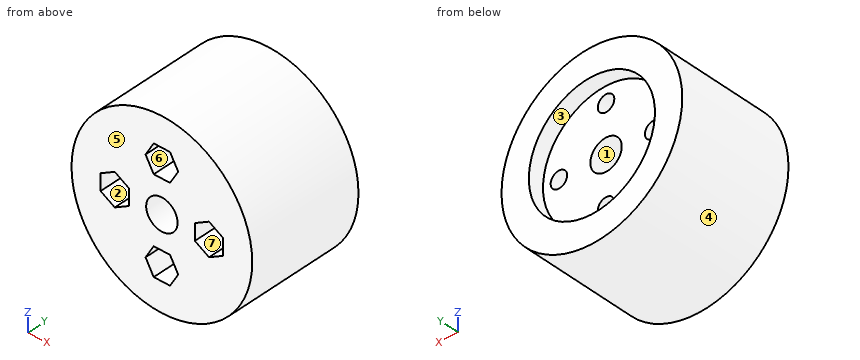
from build123d import *

# Parameters (mm, degrees)
SKETCH1_R           = 23
SKETCH1_R_2         = 4
SKETCH1_R_3         = 2.1
BOSS_EXTRUDE1_DEPTH = 30
SKETCH2_R           = 16.05
CUT_EXTRUDE1_DEPTH  = 4
CUT_EXTRUDE2_DEPTH  = 12


with BuildPart() as part:
    # Sketch1 → Boss-Extrude1 (new body)
    with BuildSketch(Plane(origin=(0, 0, 0), x_dir=(1, 0, 0), z_dir=(0, 1, 0))):
        with Locations(Location((0, 0, 0), (0, 0, 270))):
            Circle(SKETCH1_R)
        with Locations(Location((0, 0, 0), (0, 0, 270))):
            Circle(SKETCH1_R_2, mode=Mode.SUBTRACT)
        with Locations(Location((0, 12, 0), (0, 0, 270))):
            Circle(SKETCH1_R_3, mode=Mode.SUBTRACT)
        with Locations(Location((12, 0, 0), (0, 0, 270))):
            Circle(SKETCH1_R_3, mode=Mode.SUBTRACT)
        with Locations(Location((0, -12, 0), (0, 0, 270))):
            Circle(SKETCH1_R_3, mode=Mode.SUBTRACT)
        with Locations(Location((-12, 0, 0), (0, 0, 270))):
            Circle(SKETCH1_R_3, mode=Mode.SUBTRACT)
    extrude(amount=BOSS_EXTRUDE1_DEPTH)

    # Sketch2 → Cut-Extrude1 (cut)
    with BuildSketch(Plane(origin=(0, 30, 0), x_dir=(1, 0, 0), z_dir=(0, 1, 0))):
        with Locations(Location((0, 0, 0), (0, 0, 270))):
            Circle(SKETCH2_R)
    extrude(amount=-CUT_EXTRUDE1_DEPTH, mode=Mode.SUBTRACT)

    # Sketch3 → Cut-Extrude2 (cut)
    with BuildSketch(Plane.XZ):
        Polygon((12, -4.156921938), (15.6, -2.078460969), (15.6, 2.078460969), (12, 4.156921938), (8.4, 2.078460969), (8.4, -2.078460969), align=None)
        Polygon((4.156921938, 12), (2.078460969, 15.6), (-2.078460969, 15.6), (-4.156921938, 12), (-2.078460969, 8.4), (2.078460969, 8.4), align=None)
        Polygon((-4.156921938, -12), (-2.078460969, -15.6), (2.078460969, -15.6), (4.156921938, -12), (2.078460969, -8.4), (-2.078460969, -8.4), align=None)
        Polygon((-12, 4.156921938), (-15.6, 2.078460969), (-15.6, -2.078460969), (-12, -4.156921938), (-8.4, -2.078460969), (-8.4, 2.078460969), align=None)
    extrude(amount=-CUT_EXTRUDE2_DEPTH, mode=Mode.SUBTRACT)


solid = part.part
Build history of the part. All positions in model axes, mm. Face numbers are marked on the shaded views. A direction names the side the tool comes from. Coordinates: 2 decimals unless noted, no trailing zeros. Order: outer loops, then holes, each group sorted by start corner. A loop starts at its lowest first (then second) coordinate and runs counter-clockwise, first axis right, second up. Notation, with made-up numbers: (-38, -9) - (-4, -9) arc R26 ccw to (-4, 22) - close; hole circle Ø5 at (55, 75.5). An arc over 180 degrees is marked (long way). Write each question's results on one line, items separated by ' | '. Start each with the question number.
Item 1: Flat gauge pins, fed straight in: pin 1 (4 mm diameter, centred on y = 21.5, z = -10, fed in from +X); pin 2 (2 mm diameter, centred on x = 1.5, z = -13, fed in from -Y); pin 3 (12 mm diameter, centred on y = 5, z = -1.5, fed in from +X); pin 4 (1.5 mm diameter, centred on x = -0.5, z = -13, fed in from -Y). Where does each tip first touch, or does it go through?
Item 2: Tool access for the marked faces 1, 2 and 3: list every direction of +Z, -Z, +X, -X, +Y, -Y with a clear straight run to the whole face (end or side of a thin tool).
Item 3: Band-saw the part on D-D on z = -13.5. Write the cut outline in (x, y).
Item 4: Band-saw the part on C-C on y = 2.5. Write the cut outline in (x, z).
Item 5: Band-saw the part on A-A on x = 0. Write the cut outline in (y, z), and give its area (3 significant figures).
Item 6: Mould opens along Z. For the marked faces 4, 5, 6 and 7 say: released by +Z, released by -Z, zero draft, split by the parting line, or undercut.
Item 7: Band-saw the part on B-B on z = 0. Write the cut outline in (x, y), and give its area (3 significant figures).
Item 8: Wall check: probe 1 along X at (y, z) = (13.5, 0); probe 2 along X at (y, z) = (6.5, 3.5); probe 3 along Y at (x, z) = (2.5, -8). Give the ranges that are in metal, low to high. Write a range as [from, to].
Numbers:
1) pin 1: x = 21.56 | pin 2: y = 12 | pin 3: x = 23 | pin 4: through
2) face 1: +Y, -Y | face 2: -Y | face 3: +Y
3) outline: (-18.62, 0) - (-3.29, 0) - (-3.29, 12) - (-1.47, 12) - (-1.47, 26) - (-8.68, 26) - (-8.68, 30) - (-18.62, 30) - close; (1.47, 12) - (3.29, 12) - (3.29, 0) - (18.62, 0) - (18.62, 30) - (8.68, 30) - (8.68, 26) - (1.47, 26) - close
4) outline: circle Ø46 at (0, 0); hole (-15.6, -2.08) - (-12, -4.16) - (-8.4, -2.08) - (-8.4, 2.08) - (-12, 4.16) - (-15.6, 2.08) - close; hole (-4.16, -12) - (-2.08, -15.6) - (2.08, -15.6) - (4.16, -12) - (2.08, -8.4) - (-2.08, -8.4) - close; hole (-4.16, 12) - (-2.08, 8.4) - (2.08, 8.4) - (4.16, 12) - (2.08, 15.6) - (-2.08, 15.6) - close; hole circle Ø8 at (0, 0); hole (8.4, -2.08) - (12, -4.16) - (15.6, -2.08) - (15.6, 2.08) - (12, 4.16) - (8.4, 2.08) - close
5) outline: (0, -23) - (30, -23) - (30, -16.05) - (26, -16.05) - (26, -14.1) - (12, -14.1) - (12, -15.6) - (0, -15.6) - close; (0, -8.4) - (12, -8.4) - (12, -9.9) - (26, -9.9) - (26, -4) - (0, -4) - close; (0, 4) - (26, 4) - (26, 9.9) - (12, 9.9) - (12, 8.4) - (0, 8.4) - close; (0, 15.6) - (12, 15.6) - (12, 14.1) - (26, 14.1) - (26, 16.05) - (30, 16.05) - (30, 23) - (0, 23) - close | area: 753 mm^2
6) face 4: split by the parting line | face 5: zero draft | face 6: undercut | face 7: undercut
7) outline: (-23, 0) - (-15.6, 0) - (-15.6, 12) - (-14.1, 12) - (-14.1, 26) - (-16.05, 26) - (-16.05, 30) - (-23, 30) - close; (-9.9, 12) - (-8.4, 12) - (-8.4, 0) - (-4, 0) - (-4, 26) - (-9.9, 26) - close; (4, 0) - (8.4, 0) - (8.4, 12) - (9.9, 12) - (9.9, 26) - (4, 26) - close; (14.1, 12) - (15.6, 12) - (15.6, 0) - (23, 0) - (23, 30) - (16.05, 30) - (16.05, 26) - (14.1, 26) - close | area: 753 mm^2
8) probe 1: [-23, -14.1], [-9.9, -4], [4, 9.9], [14.1, 23] | probe 2: [-22.73, -13.14], [-10.86, -1.94], [1.94, 10.86], [13.14, 22.73] | probe 3: [0, 26]
